The model under review builds one solid part; all positions refer to its coordinate system, in mm. Coordinates: 2 decimals unless noted, no trailing zeros. Write each loop counter-clockwise with the first axis right and the second up, starting at its lowest first coordinate (ties: lowest second). Pieces come first, ordered by that corner, then holes.
1) Mouldability with a two-part tool opening along X and no side actions: class faces 1 (the flat face through (0, 3, 2)), 2 (the flat face through (-30, -6, 1)), 3 (the cylindrical face through (23.82, -3.92, 0.99)) as released by +X, released by -X, zero draft, split by the parting line, or undercut.
2) Add section C-C, the plane x = 25. State the section outline as (y, z) points.
3) For line 1 (X direction, y = -5, z = 0.95); line 2 (Y direction, x = 25, z = 0.8); line 3 (X direction, y = 22.5, z = 1.15), list the stretches that pass through material, from the lowest coordinate up.
4) Add section A-A, the plane y = -5. State the section outline as (x, z) points, then the cut area to 3 significant figures.
5) Add section D-D, the plane x = -17.5. State the section outline as (y, z) points, then the cut area to 3 significant figures.
6) Add section B-B, the plane z = 1.35. State the section outline as (x, y) points.
from build123d import *

# Parameters (mm, degrees)
EXTRUDE_367_DEPTH          = 2
CUT_EXTRUDE_570_DEPTH      = 41.410394702
CUT_EXTRUDE_570_DEPTH_BACK = 41.410394702
SKETCH_2_R                 = 1.6
FILLET_1_R                 = 1


with BuildPart() as part:
    # Эскиз1 → Extrude 367 (new body)
    with BuildSketch(Plane.XY):
        with BuildLine():
            Line((-30, 0), (-30, -12.5))
            Line((-30, -12.5), (30, -12.5))
            Line((30, -12.5), (30, 0))
            ThreePointArc((30, 0), (0, 27), (-30, 0))
        make_face()
    extrude(amount=EXTRUDE_367_DEPTH)

    # Эскиз2 → Cut-Extrude 570 (cut, two sides: drawn at the far end of the back side and taken through both)
    with BuildSketch(Plane.XY.offset(2).offset(-CUT_EXTRUDE_570_DEPTH_BACK)):
        with Locations((-25, -5)):
            Circle(SKETCH_2_R)
        with Locations((25, -5)):
            Circle(SKETCH_2_R)
    extrude(amount=CUT_EXTRUDE_570_DEPTH + CUT_EXTRUDE_570_DEPTH_BACK, mode=Mode.SUBTRACT)

    # Скругление1
    fillet_1_edges = [part.edges().sort_by_distance(p)[0] for p in [
        (30, 0, 1),
        (30, -12.5, 1),
        (-30, -12.5, 1),
        (-30, 0, 1),
    ]]
    fillet(fillet_1_edges, radius=FILLET_1_R)


solid = part.part
Geometry results:
1. face 1: zero draft
1. face 2: released by -X
1. face 3: undercut
2. outline: (-12.5, 0) - (-6.6, 0) - (-6.6, 2) - (-12.5, 2) - close; (-3.4, 0) - (13.72, 0) - (13.72, 2) - (-3.4, 2) - close
3. line 1: x = -30 to -26.6, -23.4 to 23.4, 26.6 to 30
3. line 2: y = -12.5 to -6.6, -3.4 to 13.72
3. line 3: x = -15.85 to 15.85
4. outline: (-30, 0) - (-26.6, 0) - (-26.6, 2) - (-30, 2) - close; (-23.4, 0) - (23.4, 0) - (23.4, 2) - (-23.4, 2) - close; (26.6, 0) - (30, 0) - (30, 2) - (26.6, 2) - close
4. area: 107 mm2
5. outline: (-12.5, 0) - (21.41, 0) - (21.41, 2) - (-12.5, 2) - close
5. area: 67.8 mm2
6. outline: (-30, -11.5) arc R1 ccw to (-29, -12.5) - (29, -12.5) arc R1 ccw to (30, -11.5) - (30, -0.05) arc R1 ccw to (29.99, 0.05) arc R30.17 ccw to (-29.99, 0.05) arc R1 ccw to (-30, -0.05) - close; hole circle Ø3.2 at (-25, -5); hole circle Ø3.2 at (25, -5)
